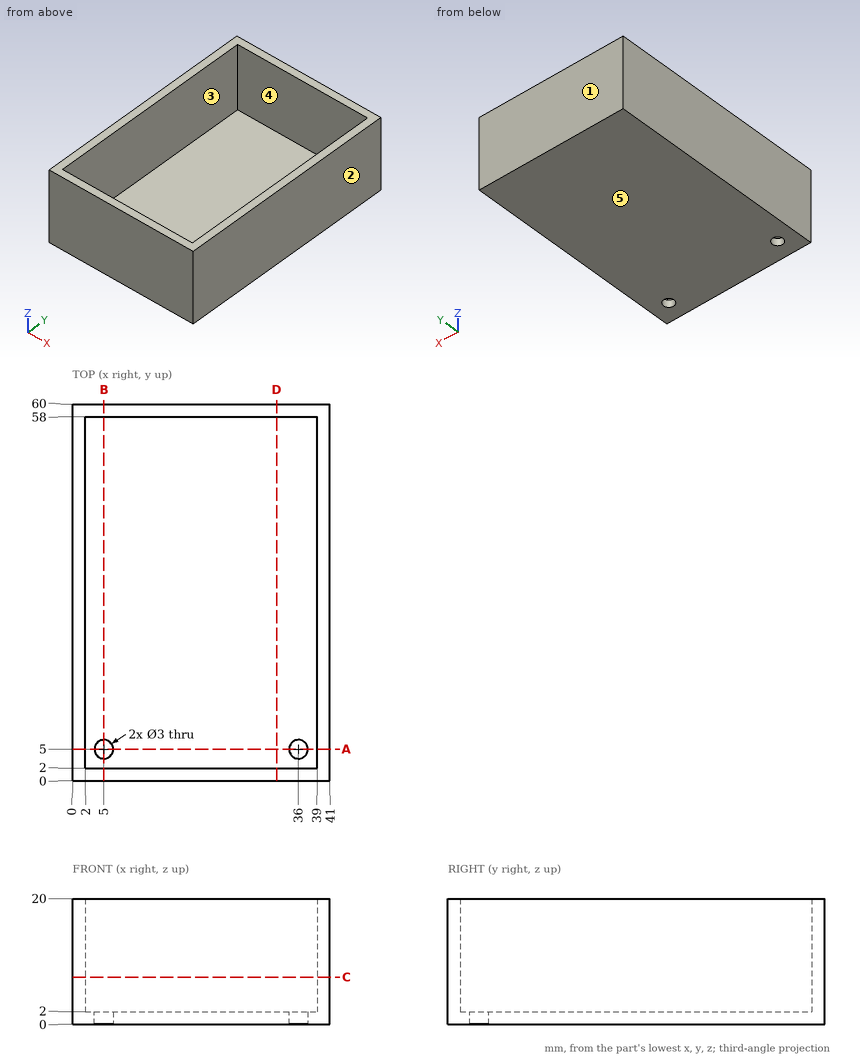
Study the drawing (mm; zero at the part's minimum x, y, z) and answer. A direction names the side the tool comes from. Coordinates: 2 decimals unless noted, no trailing zeros. Write each loop counter-clockwise with the first axis right and the second up, starting at its lowest first coordinate (ties: lowest second). Pieces come first, ordered by that corner, then holes.
Q1. Each of these flat-tipped pins is pushed along its axis until it touches: pin 1 Ø2 at (x, z) = (18, 8.5) entering from -Y; pin 2 Ø1 at (x, y) = (16.5, 48) entering from +Z. Where does it stop, or does it pass through?
Q2. Which of the six approach directions +Z, -Z, +X, -X, +Y, -Y give full straight-line access (tool end or side, diameter ignored) to the marked faces 4 and 5?
Q3. A cutting plane is placed at D-D, the plane x = 32.5. Give the vertices of the cut face in (y, z), then the cut area to 3 significant figures.
Q4. A cutting plane is placed at C-C, the plane z = 7.5. Give the vertices of the cut face in (x, y).
Q5. Determine the mould class of the marked faces 1, 2 and 3 for opening direction X: released by +X, released by -X, zero draft, split by the parting line, or undercut.
Q6. A cutting plane is placed at B-B, the plane x = 5. Give the vertices of the cut face in (y, z), then the cut area to 3 significant figures.
Q7. A cutting plane is placed at A-A, the plane y = 5. Give the vertices of the cut face in (x, z), then the cut area to 3 significant figures.
Q8. Find the intervals of material crossed by line 1 (Y direction, x = 16, z = 8.25); line 2 (X direction, y = 21.5, z = 11.5); line 3 (Y direction, x = 36, z = 0.6), in increasing order.
Findings below:
1. pin 1: stops at y = 0
1. pin 2: stops at z = 2
2. face 4: +Z
2. face 5: -Z, +X, -X, +Y, -Y
3. outline: (0, 0) - (60, 0) - (60, 20) - (58, 20) - (58, 2) - (2, 2) - (2, 20) - (0, 20) - close
3. area: 192 mm2
4. outline: (0, 0) - (41, 0) - (41, 60) - (0, 60) - close; hole (2, 2) - (39, 2) - (39, 58) - (2, 58) - close
5. face 1: zero draft
5. face 2: released by +X
5. face 3: undercut
6. outline: (0, 0) - (3.5, 0) - (3.5, 2) - (2, 2) - (2, 20) - (0, 20) - close; (6.5, 0) - (60, 0) - (60, 20) - (58, 20) - (58, 2) - (6.5, 2) - close
6. area: 186 mm2
7. outline: (0, 0) - (3.5, 0) - (3.5, 2) - (2, 2) - (2, 20) - (0, 20) - close; (6.5, 0) - (34.5, 0) - (34.5, 2) - (6.5, 2) - close; (37.5, 0) - (41, 0) - (41, 20) - (39, 20) - (39, 2) - (37.5, 2) - close
7. area: 142 mm2
8. line 1: y = 0 to 2, 58 to 60
8. line 2: x = 0 to 2, 39 to 41
8. line 3: y = 0 to 3.5, 6.5 to 60
